Build history of the part. All positions in model axes, mm. Give positions to 0.01 mm unless a question says otherwise; leave off trailing zeros. Loops run counter-clockwise (first coordinate to the right, second up) from the corner with the lowest first, then second, coordinate; pieces in that order, holes last.
1) Band-saw the part on A-A on y = 0. List the corners of the cut face in (x, z), then the cut area to 3 significant figures.
2) Two-plate mould, pull along Y, no slides. Class faces 1 (the flat face through (1, 0, -81.25)), 2 (the flat face through (1, -15, -40)), 3 (the cylindrical face through (1.48, -0.09, -74.15)): +Y half, -Y half, draft (parallel to the pull), parting line (faces both ways), or undercut.
3) Flat gauge pins, fed straight in: P1, Ø4, axis at y = 10.39, z = 6, coming from the -X side; P2, Ø1, axis at x = 0.5, y = 6, coming from the +Z side. Where does each tip first touch, or does it go through?
4) Band-saw the part on B-B on z = -12. List the corners of the cut face in (x, y), then the cut area to 3 significant figures.
5) Wall check: line 1 (Z direction, x = 1.6, y = 0); line 2 (Y direction, x = 1.3, z = -46.25); line 3 (Y direction, x = 0.8, z = -6). Give the ranges that are in metal, low to high.
6) Band-saw the part on C-C on y = -9.5. List the corners of the cut face in (x, z).
7) Band-saw the part on D-D on z = 7. List the corners of the cut face in (x, y).
Autodesk Inventor part; units mm, degrees
ref_plane "YZ Plane" through (0, 0, 0) normal (1, 0, 0) x (0, 1, 0)
ref_plane "XZ Plane" through (0, 0, 0) normal (0, 1, 0) x (-1, 0, 0)
ref_plane "XY Plane" through (0, 0, 0) normal (0, 0, 1) x (1, 0, 0)
sketch "スケッチ1" plane through (0, 0, 0) normal (1, 0, 0) x (0, 1, 0)
  circle A0 centre (0, 0) radius 15
  line L0 (15, -41.25) -> (-15, -41.25)
  line L1 (-15, -41.25) -> (-15, -81.25)
  line L2 (-15, -81.25) -> (15, -81.25)
  line L3 (15, -81.25) -> (15, -41.25)
  line L4 (15, -41.25) -> (15, 0)
  line L5 (-15, 0) -> (-15, -41.25)
  dimension "d0" = 30
  dimension "d1" = 30
  dimension "d2" = 40
  dimension "d4" = 15
  dimension "d28" = 41.25
extrude "押し出し1" add sketch "スケッチ1" along normal blind 3
sketch "スケッチ2" plane through (3, 0, 0) normal (1, 0, 0) x (0, 0, -1)
  circle A0 centre (0, 0) radius 12
  line L0 (81.25, 15) -> (0, 15)
  line L1 (81.25, -15) -> (81.25, 15)
  point P0 (12, 0)
  point P1 (6, 10.3923)
  point P2 (-6, 10.3923)
  point P3 (-12, 0)
  point P4 (-6, -10.3923)
  point P5 (6, -10.3923)
  dimension "d7" = 24
  dimension "d10" = 360
hole "穴1" at (3, 0, -12) at (3, 10.3923, -6) at (3, 10.3923, 6) at (3, 0, 12) at (3, -10.3923, 6) at (3, -10.3923, -6) direction (-1, 0, 0) diameter 4.2 end through all
sketch "スケッチ5" plane through (3, 0, 0) normal (1, 0, 0) x (0, 0, -1)
  line L0 (81.25, -15) -> (81.25, 15)
  point P0 (0, 0)
  point P1 (76.25, 0)
  point P2 (46.25, 0)
  dimension "d40" = 5
  dimension "d41" = 30
hole "穴3" at (3, 0, -76.25) at (3, 0, -46.25) direction (-1, 0, 0) diameter 4.2 end through all
properties part number "link4_plate4" material "アルミニウム 6061"
Findings below:
1. outline: (0, -81.25) - (3, -81.25) - (3, -78.35) - (0, -78.35) - close; (0, -74.15) - (3, -74.15) - (3, -48.35) - (0, -48.35) - close; (0, -44.15) - (3, -44.15) - (3, -14.1) - (0, -14.1) - close; (0, -9.9) - (3, -9.9) - (3, 9.9) - (0, 9.9) - close; (0, 14.1) - (3, 14.1) - (3, 15) - (0, 15) - close
1. area: 238 mm2
2. face 1: draft
2. face 2: -Y half
2. face 3: undercut
3. P1: passes through
3. P2: stops at z = 13.96
4. outline: (0, -15) - (3, -15) - (3, -2.1) - (0, -2.1) - close; (0, 2.1) - (3, 2.1) - (3, 15) - (0, 15) - close
4. area: 77.4 mm2
5. line 1: z = -81.25 to -78.35, -74.15 to -48.35, -44.15 to -14.1, -9.9 to 9.9, 14.1 to 15
5. line 2: y = -15 to -2.1, 2.1 to 15
5. line 3: y = -15 to -12.49, -8.29 to 8.29, 12.49 to 15
6. outline: (0, -81.25) - (3, -81.25) - (3, -7.9) - (0, -7.9) - close; (0, -4.1) - (3, -4.1) - (3, 4.1) - (0, 4.1) - close; (0, 7.9) - (3, 7.9) - (3, 11.61) - (0, 11.61) - close
7. outline: (0, -13.27) - (3, -13.27) - (3, -12.24) - (0, -12.24) - close; (0, -8.55) - (3, -8.55) - (3, 8.55) - (0, 8.55) - close; (0, 12.24) - (3, 12.24) - (3, 13.27) - (0, 13.27) - close
